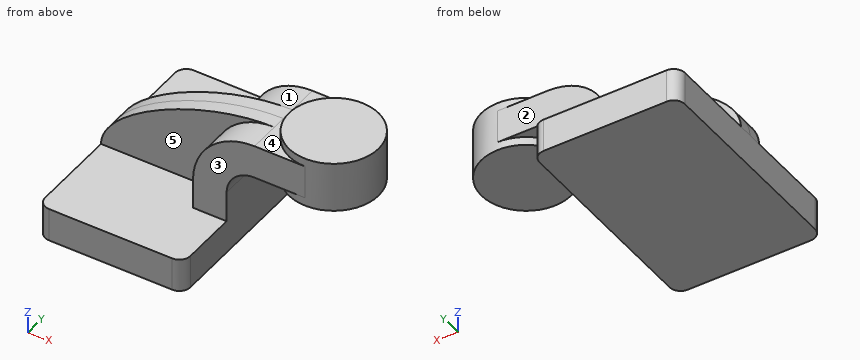
```python
from build123d import *

# Parameters (mm, degrees)
F1_DEPTH = 63.5
F0_W     = 25.4
F0_H     = 19.05
F2_DEPTH = 25.4
F4_DEPTH = 7.9375
F5_R     = 6.35


with BuildPart() as f1:
    # F0 (on Front) → F1 (new body, symmetric)
    with BuildSketch(Plane.XZ):
        Polygon((41.275, -9.525), (41.275, 9.525), (22.225, 9.525), (-41.275, 9.525), (-41.275, -9.525), align=None)
    extrude(amount=F1_DEPTH, both=True)

    # F0 (on Front) → F2 (join, symmetric)
    with BuildSketch(Plane.XZ):
        with BuildLine():
            Line((22.225, 9.525), (41.275, 9.525))
            Line((41.275, 9.525), (41.275, 26.9875))
            ThreePointArc((41.275, 26.9875), (45.9246798487, 38.2128201513), (57.15, 42.8625))
            Line((57.15, 42.8625), (60.325, 42.8625))
            Line((60.325, 42.8625), (60.325, 61.9125))
            Line((60.325, 61.9125), (57.15, 61.9125))
            ThreePointArc((57.15, 61.9125), (32.4542956671, 51.6832043329), (22.225, 26.9875))
            Line((22.225, 26.9875), (22.225, 9.525))
        make_face()
        with Locations((73.025, 52.3875)):
            Rectangle(F0_W, F0_H)
    extrude(amount=F2_DEPTH, both=True)

    # F0 (on Front) → F3 (revolve)
    with BuildSketch(Plane.XZ):
        Polygon((85.725, 61.9125), (85.725, 42.8625), (85.725, 38.1), (111.125, 38.1), (111.125, 66.675), (85.725, 66.675), align=None)
    revolve(axis=Axis((85.725, 0, 52.3875), (0, 0, 1)))

    # F0 (on Front) → F4 (join, symmetric)
    with BuildSketch(Plane.XZ):
        with BuildLine():
            Line((-41.275, 9.525), (22.225, 9.525))
            Line((22.225, 9.525), (22.225, 26.9875))
            ThreePointArc((22.225, 26.9875), (32.4542956671, 51.6832043329), (57.15, 61.9125))
            add(Edge.make_bspline(
                [(-41.275, 9.525), (-41.275, 33.1159606576), (15.4643859714, 61.9125), (57.15, 61.9125)],
                knots=[0, 0, 0, 0, 111.4985685166, 111.4985685166, 111.4985685166, 111.4985685166], degree=3))
        make_face()
    extrude(amount=F4_DEPTH, both=True)

    # F5
    f5_edges = [f1.edges().sort_by_distance(p)[0] for p in [
        (-41.275, -63.5, 0),
        (41.275, -63.5, 0),
        (-41.275, 63.5, 0),
        (41.275, 63.5, 0),
    ]]
    fillet(f5_edges, radius=F5_R)


solid = f1.part
```
Check sheet for the modelled part. Datum: model origin and axes. Units: mm. Face numbers are marked on the shaded views. A direction names the side the tool comes from. Coordinates: 2 decimals unless noted, no trailing zeros. Loops run counter-clockwise (first coordinate to the right, second up) from the corner with the lowest first, then second, coordinate; pieces in that order, holes last.
1) Gauge pin test, flat ends, axial feed: pin 1 (15.5 mm diameter, centred on x = 12, z = 33, fed in from -Y); pin 2 (5 mm diameter, centred on x = 81.5, y = -12.5, fed in from -Z); pin 3 (10 mm diameter, centred on x = 12, y = 28.5, fed in from +Z) (3 decimals). Record the tip position at first contact, or that the pin passes through.
2) Access from +Z, -Z, +X, -X, +Y, -Y to the whole of each face (thin tool, end or side, straight path). Record for the marked faces 1, 2, 3, 4 and 5.
3) Sectioned sample at A-A (x = 80). Record the boundary of the cut face in (y, z) (1 decimal), and give its area (3 significant figures).
4) Material ranges on probe 1 along X at (y, z) = (54.5, 6.5) (3 decimals); probe 2 along Z at (x, y) = (-29, 26) (3 decimals); probe 3 along Y at (x, z) = (38.5, 21.5), recorded low to high.
5) Sectioned sample at B-B (y = 31.5). Record the boundary of the cut face in (x, z) (3 decimals), and give its area (3 significant figures).
Check sheet entries:
1. pin 1: stops at y = -7.94
1. pin 2: stops at z = 38.1
1. pin 3: stops at z = 9.525
2. face 1: +Z, -X, +Y
2. face 2: +Z, +X, -X, +Y
2. face 3: +Z, +X, -X, -Y
2. face 4: +Z, -X
2. face 5: +Z, -X, -Y
3. outline: (-25.4, 42.9) - (-24.7, 42.9) - (-24.7, 38.1) - (24.7, 38.1) - (24.7, 42.9) - (25.4, 42.9) - (25.4, 61.9) - (24.7, 61.9) - (24.7, 66.7) - (-24.7, 66.7) - (-24.7, 61.9) - (-25.4, 61.9) - close
3. area: 1,440 mm2
4. probe 1: x = -41.275 to 41.275
4. probe 2: z = -9.525 to 9.525
4. probe 3: y = -25.4 to 25.4
5. outline: (-41.275, -9.525) - (41.275, -9.525) - (41.275, 9.525) - (-41.275, 9.525) - close
5. area: 1,570 mm2
